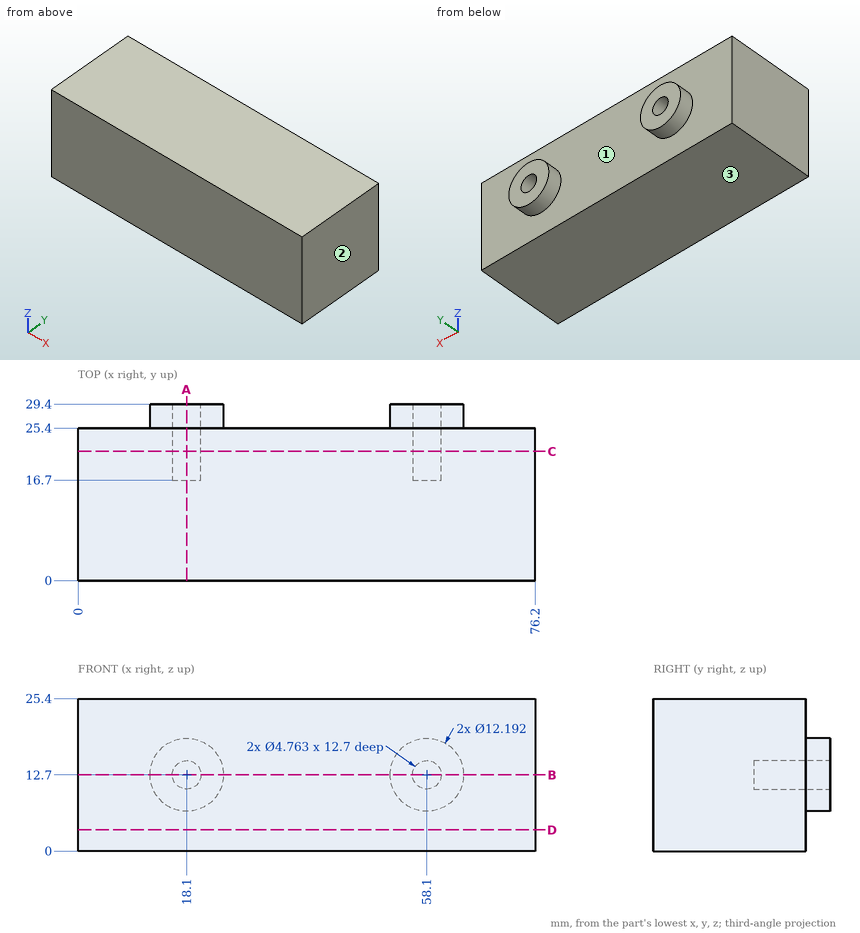
Check sheet for the drawn part. Datum: minimum x, y, z corner. Units: mm. Round coordinates to 2 decimals unless told otherwise and drop trailing zeros. Loops run counter-clockwise (first coordinate to the right, second up) from the corner with the lowest first, then second, coordinate; pieces in that order, holes last. Notation, with made-up numbers: (-26.5, 25.25) - (-21.5, 25.25) arc R25 ccw to (-21.5, 42.25) - close; hole circle Ø8 at (-8.75, -36). An arc over 180 degrees is marked (long way). Use one line per item in the form item = value.
1. Section check C-C on y = 21.5. Record the cut outline in (x, z), and give its area (3 significant figures).
A:
outline = (0, 0) - (76.2, 0) - (76.2, 25.4) - (0, 25.4) - close; hole circle Ø4.76 at (18.1, 12.7); hole circle Ø4.76 at (58.1, 12.7)
area = 1,900 mm²
2. Gauge pin test, flat ends, axial feed: pin 1 Ø10 at (x, z) = (43, 4.5) entering from +Y; pin 2 Ø3 at (x, z) = (58.1, 12.7) entering from +Y. Record the tip position at first contact, or that the pin passes through.
A:
pin_1 = 25.4
pin_2 = 16.7
3. Section check D-D on z = 3.5. Record the cut outline in (x, y), and give its area (3 significant figures).
A:
outline = (0, 0) - (76.2, 0) - (76.2, 25.4) - (0, 25.4) - close
area = 1,940 mm²
4. Draft check along X on the marked faces 1, 2 and 3. Enter one of: pulls with the +X half, pulls with the -X half, needs draft (parallel to the pull), parting line crosses it, or undercut.
A:
face_1 = undercut
face_2 = pulls with the +X half
face_3 = needs draft
5. Scan lines: probe 1 along Z at (x, y) = (18.1, 22); probe 2 along X at (y, z) = (19.75, 13.5); probe 3 along Z at (x, y) = (18.1, 26.5). Record each from-to range of solid material in increasing order.
A:
probe_1 = 0 to 10.32, 15.08 to 25.4
probe_2 = 0 to 15.86, 20.34 to 55.86, 60.34 to 76.2
probe_3 = 6.6 to 10.32, 15.08 to 18.8
6. Section check A-A on x = 18.1. Record the cut outline in (y, z).
A:
outline = (0, 0) - (25.4, 0) - (25.4, 6.6) - (29.4, 6.6) - (29.4, 10.32) - (16.7, 10.32) - (16.7, 15.08) - (29.4, 15.08) - (29.4, 18.8) - (25.4, 18.8) - (25.4, 25.4) - (0, 25.4) - close
7. Section check B-B on z = 12.7. Record the cut outline in (x, y).
A:
outline = (0, 0) - (76.2, 0) - (76.2, 25.4) - (64.2, 25.4) - (64.2, 29.4) - (60.48, 29.4) - (60.48, 16.7) - (55.72, 16.7) - (55.72, 29.4) - (52, 29.4) - (52, 25.4) - (24.2, 25.4) - (24.2, 29.4) - (20.48, 29.4) - (20.48, 16.7) - (15.72, 16.7) - (15.72, 29.4) - (12, 29.4) - (12, 25.4) - (0, 25.4) - close
